Part print with two shaded views. Sizes in mm from the minimum x, y, z corner. Round coordinates to 2 decimals unless told otherwise and drop trailing zeros. Loops run counter-clockwise (first coordinate to the right, second up) from the corner with the lowest first, then second, coordinate; pieces in that order, holes last. Notation, with made-up numbers: (55.5, -16.75) -> (71.5, -16.75) arc R17 cw to (71.5, 15.25) -> close; hole circle Ø4 at (47, -9). An arc over 180 degrees is marked (long way). Use a Markdown table: item, result. Add a question column.
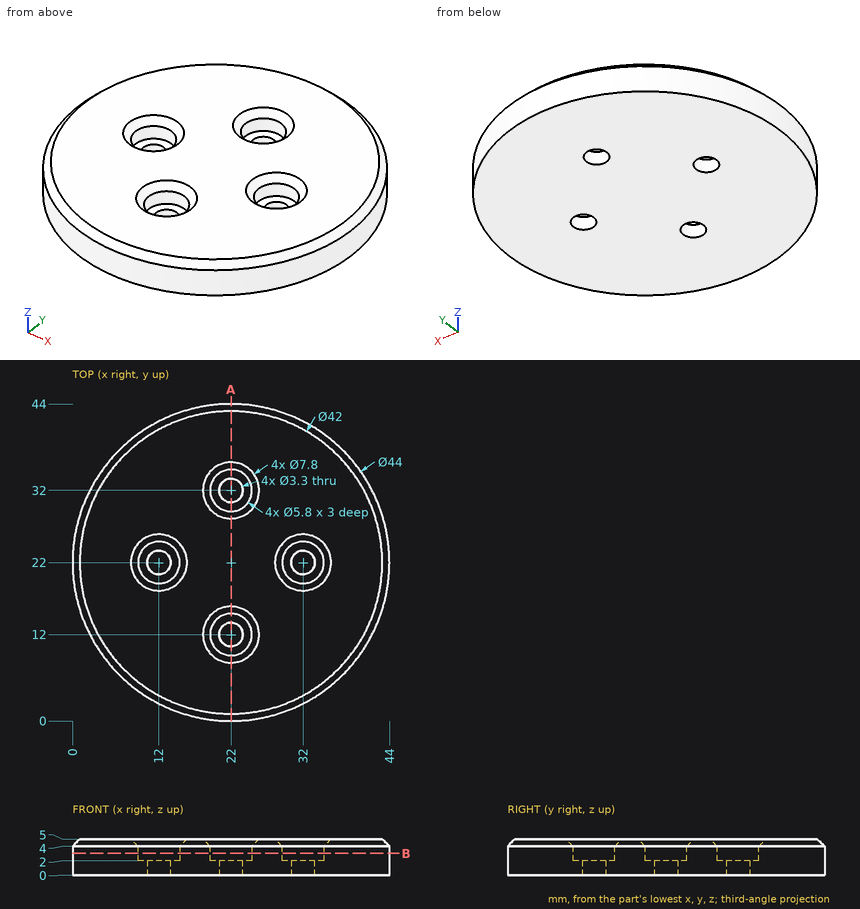
1) Wall check: probe 1 along Y at (x, z) = (22, 3.6); probe 2 along Y at (x, z) = (32, 3.25); probe 3 along X at (y, z) = (12, 0.55). Give the ranges that are in metal, low to high. Write a range as from..to.
2) Cut at A-A on x = 22. Write the cut outline in (y, z).
3) Pin check, flat tips, straight feed: pin 1 Ø1 at (x, y) = (21, 11) entering from +Z; pin 2 Ø1.5 at (x, z) = (28, 1.5) entering from -Y; pin 3 Ø6.5 at (x, y) = (12, 22) entering from +Z. Stop position of each tip, or through.
4) Cut at B-B on z = 3. Write the cut outline in (x, y), and give its area (3 significant figures).
Established:
| question | item | result |
|---|---|---|
| 1 | probe 1 | y = 0..9.1, 14.9..29.1, 34.9..44 |
| 1 | probe 2 | y = 2.4..19.1, 24.9..41.6 |
| 1 | probe 3 | x = 2.4..20.35, 23.65..41.6 |
| 2 | outline | (0, 0) -> (10.35, 0) -> (10.35, 2) -> (9.1, 2) -> (9.1, 4) -> (8.1, 5) -> (1, 5) -> (0, 4) -> close; (13.65, 0) -> (30.35, 0) -> (30.35, 2) -> (29.1, 2) -> (29.1, 4) -> (28.1, 5) -> (15.9, 5) -> (14.9, 4) -> (14.9, 2) -> (13.65, 2) -> close; (33.65, 0) -> (44, 0) -> (44, 4) -> (43, 5) -> (35.9, 5) -> (34.9, 4) -> (34.9, 2) -> (33.65, 2) -> close |
| 3 | pin 1 | stops at z = 2 |
| 3 | pin 2 | stops at y = 0.64 |
| 3 | pin 3 | stops at z = 4.35 |
| 4 | outline | circle Ø44 at (22, 22); hole circle Ø5.8 at (12, 22); hole circle Ø5.8 at (22, 12); hole circle Ø5.8 at (22, 32); hole circle Ø5.8 at (32, 22) |
| 4 | area | 1,410 mm^2 |
